Can you work these out from the model? Positions are in its coordinate system, mm. A direction names the side the tool comes from. Round coordinates to 2 decimals unless told otherwise and drop trailing zeros. Write each loop counter-clockwise with the first axis right and the second up, starting at its lowest first coordinate (ties: lowest second). Pieces come first, ordered by that corner, then holes. Notation, with made-up numbers: (-14.5, -7) -> (31.5, -7) arc R29 ccw to (31.5, 23) -> close; hole circle Ø9 at (-21.5, -24.75). An arc over 180 degrees is marked (long way). Use CSV: the item, a comma, the result in double quotes.
```python
from build123d import *

# Parameters (mm, degrees)
SFAZOWANIE2_SIZE           = 1
WYTNIJ_WYCI_GNI_CIE1_DEPTH = 5.5
WYTNIJ_WYCI_GNI_CIE2_DEPTH = 6
SFAZOWANIE3_SIZE           = 2


with BuildPart() as part:
    # Szkic1 → Obr_t1 (revolve)
    with BuildSketch(Plane(origin=(0, 0, 0), x_dir=(0, 0, -1), z_dir=(1, 0, 0))):
        Polygon((-3, -6.188308688), (-3, 99.409284105), (-10.5, 99.409284105), (-10.5, 94.409284105), (-10.15, 94.409284105), (-10.15, 93.309284105), (-10.5, 93.309284105), (-10.5, 68.309284105), (-15, 68.309284105), (-15, 43.309284105), (-13, 43.309284105), (-13, 28.309284105), (-10.5, 28.309284105), (-10.5, 15), (-13, 15), (-13, 10), (-10.5, 10), (-10.5, 4.778207376), (-9.5, 4.778207376), (-9.5, 3.660040364), (-10.5, 3.660040364), (-10.5, -5), (-9.5, -5), (-9.5, -15.9), (-9.2, -15.9), (-9.2, -17), (-9.5, -17), (-9.5, -39.5), (-9.2, -39.5), (-9.2, -40.6), (-9.5, -40.6), (-9.5, -45), (-3, -45), (-3, -6.690715895), align=None)
    revolve(axis=Axis((0, 99.409284105, 3), (0, -1, 0)))

    # Sfazowanie2
    sfazowanie2_edges = [part.edges().sort_by_distance(p)[0] for p in [
        (0, 10, -7),
        (0, 15, -4.5),
        (0, 28.309284105, -4.5),
        (0, 28.309284105, -7),
        (0, 68.309284105, -9),
        (0, 99.409284105, -4.5),
    ]]
    chamfer(sfazowanie2_edges, length=SFAZOWANIE2_SIZE)

    # Szkic2 → Wytnij-wyci_gni_cie1 (cut)
    with BuildSketch(Plane(origin=(10, 0, 0), x_dir=(0, 0, -1), z_dir=(1, 0, 0))):
        with BuildLine():
            Line((-0.5, 87.721044176), (-0.5, 77.721044176))
            ThreePointArc((-0.5, 77.721044176), (-3, 75.221044176), (-5.5, 77.721044176))
            Line((-5.5, 77.721044176), (-5.5, 87.721044176))
            ThreePointArc((-5.5, 87.721044176), (-3, 90.221044176), (-0.5, 87.721044176))
        make_face()
    extrude(amount=-WYTNIJ_WYCI_GNI_CIE1_DEPTH, mode=Mode.SUBTRACT)

    # Szkic2_4 → Wytnij-wyci_gni_cie2 (cut)
    with BuildSketch(Plane(origin=(10, 0, 0), x_dir=(0, 0, -1), z_dir=(1, 0, 0))):
        with BuildLine():
            Line((-5.5, -20.047619848), (-5.5, -35.047619848))
            ThreePointArc((-5.5, -35.047619848), (-3, -37.547619848), (-0.5, -35.047619848))
            Line((-0.5, -35.047619848), (-0.5, -20.047619848))
            ThreePointArc((-0.5, -20.047619848), (-3, -17.547619848), (-5.5, -20.047619848))
        make_face()
    extrude(amount=-WYTNIJ_WYCI_GNI_CIE2_DEPTH, mode=Mode.SUBTRACT)

    # Sfazowanie3
    sfazowanie3_edges = [part.edges().sort_by_distance(p)[0] for p in [
        (0, -45, -3.5),
    ]]
    chamfer(sfazowanie3_edges, length=SFAZOWANIE3_SIZE)


solid = part.part
```
Q1. On a 3-axis mill with a long thin cutter (end or side, diameter ignored), from which of +Z, -Z, +X, -X, +Y, -Y can I reach the whole of each face in a straight line? I mean faces 1 (the face through (-7.436, 80.634, 2.024)), 2 (the face through (0, 99.409, 3)), 3 (the face through (6.345, 4.211, 1.591)), 4 (the face through (-3, -5, -3)), 5 (the face through (5.269, -37.547, 3.055)). Say none if no direction works.
Resolved:
face 1,"+Y"
face 2,"+Z, -Z, +X, -X, +Y"
face 3,"none"
face 4,"-Y"
face 5,"+X"
Q2. Suppose I cut it at A-A (y = 23). Write out the boundary of the cut face in (x, z).
Resolved:
outline,"circle Ø15 at (0, 3)"
Q3. Suppose I cut it at C-C (y = -26.5). Write out the boundary of the cut face in (x, z).
Resolved:
outline,"(4, 0.5) -> (4, 5.5) -> (6, 5.5) arc R6.5 ccw (long way) to (6, 0.5) -> close"
Q4. Please list where these lines run through material, in increasing order: probe 1 along Y at (x, z) = (-8, 6.75); probe 2 along Y at (x, z) = (-6.5, 10.75); probe 3 along X at (y, z) = (-18.5, 1).
Resolved:
probe 1,"y = 10 to 15, 28.31 to 68.31"
probe 2,"y = 43.31 to 68.31"
probe 3,"x = -6.18 to 6.18"
Q5. If we mould it in two halves opening along Y, with no side actions, what happens to faces 6 (the face through (8, 28.309, 6.3)), 7 (the face through (0, -45, 3)), 8 (the face through (7.2, 68.309, 5.6))? For each: released by +Y, released by -Y, zero draft, split by the parting line, or undercut.
Resolved:
face 6,"undercut"
face 7,"released by -Y"
face 8,"released by +Y"
Q6. Suppose I cut it at B-B (y = -8.5). Write out the boundary of the cut face in (x, z).
Resolved:
outline,"circle Ø13 at (0, 3)"
Q7. Will these pins go through, and if not, where does the flat tip stop? P1, Ø3, axis at x = -5, y = 15.5, coming from the +Z side (3 decimals); P2, Ø0.8, axis at x = 5.5, y = 84, coming from the +Z side; P3, Ø1, axis at x = 5, y = -26.5, coming from the -Z side.
Resolved:
P1,"stops at z = 12.335"
P2,"stops at z = 8.5"
P3,"stops at z = -1.69"
